```python
from build123d import *

# Parameters (mm, degrees)
BOSS_EXTRUDE1_DEPTH = 1.8
FILLET1_R           = 3
FILLET2_R           = 3
SKETCH3_R           = 7.6
CUT_EXTRUDE1_DEPTH  = 10
SCALE1_SCALE        = 1.15


with BuildPart() as part:
    # Sketch1 → Boss-Extrude1 (new body)
    with BuildSketch(Plane(origin=(0, 0, 0), x_dir=(1, 0, 0), z_dir=(0, 1, 0))):
        Polygon((-32.5, 56.291651246), (-65, 0), (-32.5, -56.291651246), (32.5, -56.291651246), (65, 0), (32.5, 56.291651246), align=None)
        with BuildLine():
            Line((-31.098446917, 47.455472674), (-56.646868343, 3.204308711))
            Line((-56.646868343, 3.204308711), (-16.055097208, 3.204308711))
            ThreePointArc((-16.055097208, 3.204308711), (-14.178339307, 8.185868015), (-10.802561349, 12.301967686))
            Line((-10.802561349, 12.301967686), (-31.098446917, 47.455472674))
        make_face(mode=Mode.SUBTRACT)
        with BuildLine():
            Line((-56.646868343, -3.204308711), (-31.098446917, -47.455472674))
            Line((-31.098446917, -47.455472674), (-10.802561349, -12.301967686))
            ThreePointArc((-10.802561349, -12.301967686), (-14.178339307, -8.185868015), (-16.055097208, -3.204308711))
            Line((-16.055097208, -3.204308711), (-56.646868343, -3.204308711))
        make_face(mode=Mode.SUBTRACT)
        with BuildLine():
            Line((-25.548421426, -50.659781385), (3, -50.659781385))
            Line((3, -50.659781385), (25.548291416, -50.659781385))
            Line((25.548291416, -50.659781385), (5.29797501, -15.490810226))
            ThreePointArc((5.29797501, -15.490810226), (4.194244938, -15.825360977), (3.069700506, -16.08137679))
            ThreePointArc((3.069700506, -16.08137679), (-1.128661889, -16.332784913), (-5.252535858, -15.506276397))
            Line((-5.252535858, -15.506276397), (-25.548421426, -50.659781385))
        make_face(mode=Mode.SUBTRACT)
        with BuildLine():
            Line((31.098446917, -47.455472674), (56.646803338, -3.204421303))
            Line((56.646803338, -3.204421303), (16.064422686, -3.157224166))
            ThreePointArc((16.064422686, -3.157224166), (14.190323862, -8.165074976), (10.802561349, -12.301967686))
            Line((10.802561349, -12.301967686), (31.098446917, -47.455472674))
        make_face(mode=Mode.SUBTRACT)
        with BuildLine():
            Line((56.646868343, 3.204308711), (31.098511922, 47.455360082))
            Line((31.098511922, 47.455360082), (10.766447676, 12.33358606))
            ThreePointArc((10.766447676, 12.33358606), (14.166324284, 8.206643464), (16.055097208, 3.204308711))
            Line((16.055097208, 3.204308711), (56.646868343, 3.204308711))
        make_face(mode=Mode.SUBTRACT)
        with BuildLine():
            Line((25.548421426, 50.659781385), (-25.548291416, 50.659781385))
            Line((-25.548291416, 50.659781385), (-5.29797501, 15.490810226))
            ThreePointArc((-5.29797501, 15.490810226), (-0.023999578, 16.37171844), (5.252535858, 15.506276397))
            Line((5.252535858, 15.506276397), (25.548421426, 50.659781385))
        make_face(mode=Mode.SUBTRACT)
        Polygon((28.926541222, 52.315471461), (31.319181202, 51.258876955), (33.063428707, 53.207907141), (31.748792971, 55.469068546), (29.192055897, 54.917512964), align=None, mode=Mode.SUBTRACT)
        Polygon((-30.843256685, 51.208855273), (-28.731899012, 52.752645025), (-29.547684912, 55.237722767), (-32.163226, 55.229795525), (-32.963933391, 52.739818478), align=None, mode=Mode.SUBTRACT)
        Polygon((59.769797908, 1.106616188), (60.051080214, -1.493768069), (62.61111362, -2.029815626), (63.912018971, 0.239273021), (62.155989288, 2.177694486), align=None, mode=Mode.SUBTRACT)
        Polygon((30.843256685, -51.208855273), (28.731899012, -52.752645025), (29.547684912, -55.237722767), (32.163226, -55.229795525), (32.963933391, -52.739818478), align=None, mode=Mode.SUBTRACT)
        Polygon((-28.926541222, -52.315471461), (-31.319181202, -51.258876955), (-33.063428707, -53.207907141), (-31.748792971, -55.469068546), (-29.192055897, -54.917512964), align=None, mode=Mode.SUBTRACT)
        Polygon((-59.769797908, -1.106616188), (-60.051080214, 1.493768069), (-62.61111362, 2.029815626), (-63.912018971, -0.239273021), (-62.155989288, -2.177694486), align=None, mode=Mode.SUBTRACT)
    extrude(amount=BOSS_EXTRUDE1_DEPTH)

    # Fillet1
    fillet1_edges = [part.edges().sort_by_distance(p)[0] for p in [
        (32.5, 0.9, -56.291651246),
        (65, 0.9, 0),
        (32.5, 0.9, 56.291651246),
        (-32.5, 0.9, 56.291651246),
        (-65, 0.9, 0),
        (-32.5, 0.9, -56.291651246),
    ]]
    fillet(fillet1_edges, radius=FILLET1_R)

    # Fillet2
    fillet2_edges = [part.edges().sort_by_distance(p)[0] for p in [
        (5.29797501, 0.9, 15.490810226),
        (-5.252535858, 0.9, 15.506276397),
        (-25.548421426, 0.9, 50.659781385),
        (25.548291416, 0.9, 50.659781385),
        (-25.548291416, 0.9, -50.659781385),
        (-5.29797501, 0.9, -15.490810226),
        (5.252535858, 0.9, -15.506276397),
        (25.548421426, 0.9, -50.659781385),
        (31.098511922, 0.9, -47.455360082),
        (10.766447676, 0.9, -12.33358606),
        (16.055097208, 0.9, -3.204308711),
        (56.646868343, 0.9, -3.204308711),
        (56.646803338, 0.9, 3.204421303),
        (16.064422686, 0.9, 3.157224166),
        (10.802561349, 0.9, 12.301967686),
        (31.098446917, 0.9, 47.455472674),
        (-31.098446917, 0.9, 47.455472674),
        (-10.802561349, 0.9, 12.301967686),
        (-16.055097208, 0.9, 3.204308711),
        (-56.646868343, 0.9, 3.204308711),
        (-10.802561349, 0.9, -12.301967686),
        (-31.098446917, 0.9, -47.455472674),
        (-56.646868343, 0.9, -3.204308711),
        (-16.055097208, 0.9, -3.204308711),
    ]]
    fillet(fillet2_edges, radius=FILLET2_R)

    # Sketch3 → Cut-Extrude1 (cut)
    with BuildSketch(Plane(origin=(0, 3.6, 0), x_dir=(1, 0, 0), z_dir=(0, 1, 0))):
        Circle(SKETCH3_R)
    extrude(amount=-CUT_EXTRUDE1_DEPTH, mode=Mode.SUBTRACT)


with BuildPart() as part_1:
    # Scale1: scaled about (-0.010587945, 0.9, 0.004669606)
    add(part.part.scale(SCALE1_SCALE).moved(Location((0.001588192, -0.135, -0.000700441))))


solid = part_1.part
```
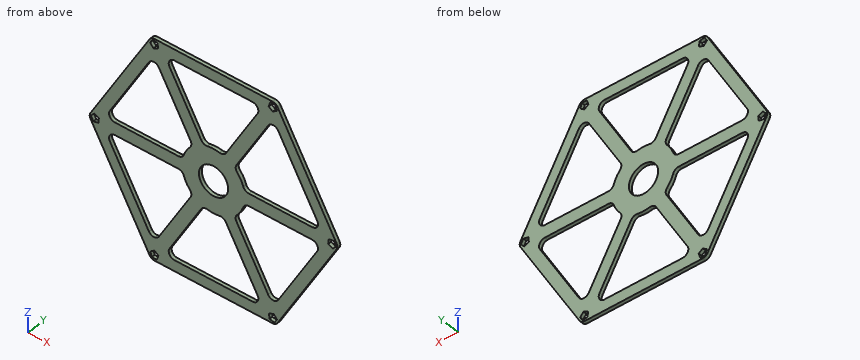
Read the model definition and answer for the solid it produces. Units are mm, in the model's axes. Give positions to 0.01 mm unless a question says otherwise; leave off trailing zeros. Write each loop counter-clockwise with the first axis right and the second up, starting at its lowest first coordinate (ties: lowest second). Pieces come first, ordered by that corner, then holes. Notation, with made-up numbers: M -26.5,48 L 31.5,48 A29 ccw 31.5,78 Z; hole C 66.5,43.5 d3. An arc over 180 degrees is marked long. Put each result on its own line as item: value. Start each with the question number.
1. The part is cut by section C-C, the plane z = 33. Give the vertices of the cut face in (x, y) (3 decimals).
2. The part is cut by section B-B, the plane z = -14.5. Give the vertices of the cut face in (x, y) (3 decimals).
3. Consider line 1 along Z through (x, y) = (54, 0.9); line 2 along Z through (x, y) = (-44, 1.05); line 3 along X through (y, z) = (0.85, 33.5). Determine where each line is inside the solid, lowest interval first.
4. Each of these flat-tipped pins is pushed along its axis until it touches: pin 1 Ø0.6 at (x, y) = (48.5, 0.5) entering from -Z; pin 2 Ø1 at (x, y) = (-39, 0.5) entering from -Z; pin 3 Ø14 at (x, z) = (0, 0) entering from -Y (3 decimals). Where does it stop, or does it pass through?
5. The part is cut by section D-D, the plane y = 0.2. Give the number of separate pieces and of enclosed holes in the cut face, and give its area (3 significant figures).
6. The part is cut by section A-A, the plane z = -55.5. Give the vertices of the cut face in (x, y) (3 decimals).
Final values:
1. outline: M -55.695,-0.135 L -48.217,-0.135 L -48.217,1.935 L -55.695,1.935 Z; M -23.306,-0.135 L -14.796,-0.135 L -14.796,1.935 L -23.306,1.935 Z; M 14.839,-0.135 L 23.31,-0.135 L 23.31,1.935 L 14.839,1.935 Z; M 48.22,-0.135 L 55.699,-0.135 L 55.699,1.935 L 48.22,1.935 Z
2. outline: M -66.377,-0.135 L -58.899,-0.135 L -58.899,1.935 L -66.377,1.935 Z; M -13.286,-0.135 L 13.256,-0.135 L 13.256,1.935 L -13.286,1.935 Z; M 58.902,-0.135 L 66.38,-0.135 L 66.38,1.935 L 58.902,1.935 Z
3. line 1: z = -35.94 to -22.99, -3.69 to 3.67, 22.99 to 35.94
3. line 2: z = -53.26 to -40.31, -3.69 to 3.68, 40.3 to 53.26
3. line 3: x = -55.41 to -47.93, -23.6 to -15.09, 15.13 to 23.6, 47.93 to 55.41
4. pin 1: stops at z = -45.99
4. pin 2: stops at z = -62.78
4. pin 3: passes through
5. separate pieces: 1
5. enclosed holes: 13
5. area: 5,740 mm²
6. outline: M -42.706,-0.135 L -26.792,-0.135 L -26.792,1.935 L -42.706,1.935 Z; M 26.787,-0.135 L 42.709,-0.135 L 42.709,1.935 L 26.787,1.935 Z
